Can you work these out from the drawing? Everything is in mm from the part's minimum corner. Round coordinates to 2 decimals unless told otherwise and drop trailing zeros. Order: outer loops, then holes, each group sorted by start corner. A loop starts at its lowest first (then second) coordinate and runs counter-clockwise, first axis right, second up. Notation, with made-up numbers: (13, 41) - (30, 41) arc R22 cw to (30, 62) - close; hole circle Ø9 at (-10.75, 8). An arc over 180 degrees is marked (long way). Write item = value, one per line.
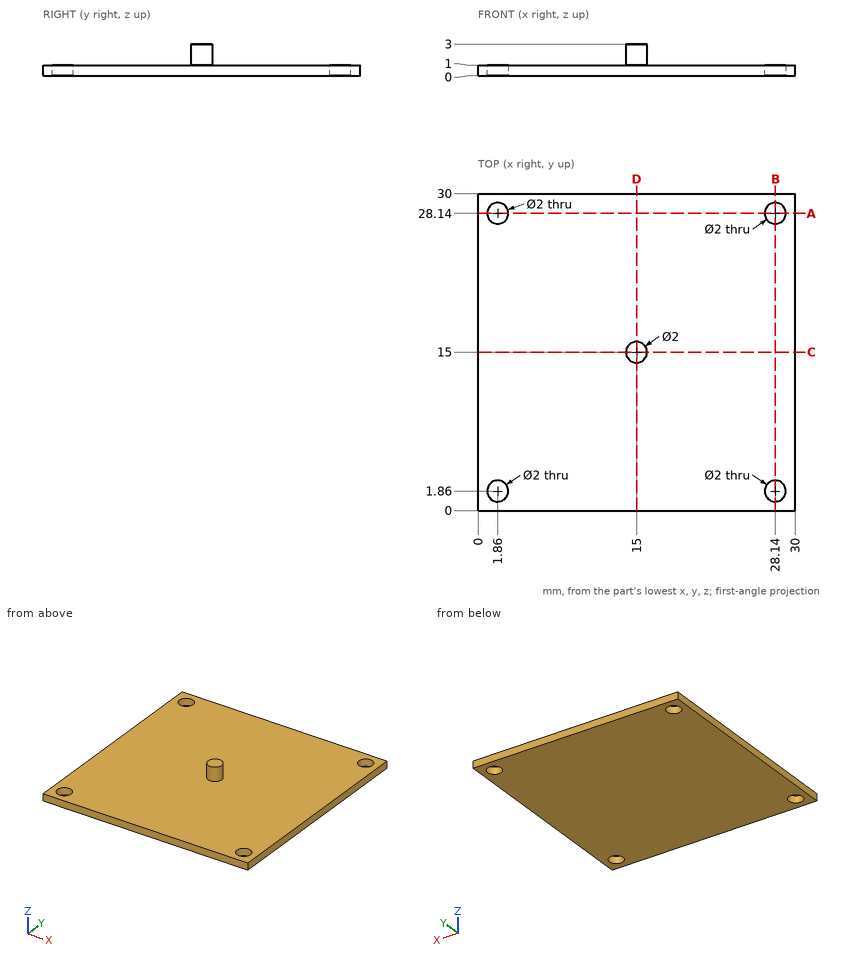
(1) If we section it at A-A (y = 28.14): Write out the boundary of the cut face in (x, z).
Computed:
outline = (0, 0) - (0.86, 0) - (0.86, 1) - (0, 1) - close; (2.86, 0) - (27.14, 0) - (27.14, 1) - (2.86, 1) - close; (29.14, 0) - (30, 0) - (30, 1) - (29.14, 1) - close
(2) If I drill on line 1 (Y direction, x = 28.14, z = 0.3); line 2 (X direction, y = 2.5, z = 0.2); line 3 (Z direction, x = 13.75, y = 9.5), over which ranges is the centre line in solid material (lowest first)? Write a range as from..to.
Computed:
line_1 = 0..0.86, 2.86..27.14, 29.14..30
line_2 = 0..1.09, 2.63..27.37, 28.91..30
line_3 = 0..1
(3) Will this pin go through, and if not, where does the flat tip stop? P1, Ø9, axis at x = 8, y = 10, coming from the +Z side.
Computed:
P1 = 1
(4) If we section it at C-C (y = 15): Write out the boundary of the cut face in (x, z).
Computed:
outline = (0, 0) - (30, 0) - (30, 1) - (16, 1) - (16, 3) - (14, 3) - (14, 1) - (0, 1) - close
